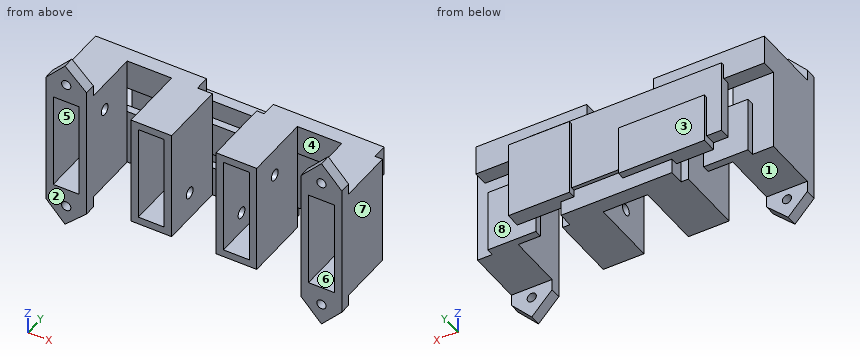
Autodesk Inventor part; units mm, degrees
ref_plane "Work Plane1" through (0, 18, 0) normal (0, 1, 0) x (-1, 0, 0)
ref_plane "YZ Plane" through (0, 0, 0) normal (1, 0, 0) x (0, 1, 0)
ref_plane "XY Plane" through (0, 0, 0) normal (0, 0, 1) x (1, 0, 0)
sketch "Sketch1" plane through (0, 0, 0) normal (0, 1, 0) x (-1, 0, 0)
  line L0 (0, 0) -> (80, 0) construction
  line L1 (80, 0) -> (80, 30) construction
  line L2 (80, 30) -> (0, 30) construction
  line L3 (0, 30) -> (0, 0) construction
  dimension "d0" = 80
  dimension "d1" = 30
sketch "Sketch2" plane through (0, 0, 0) normal (0, 1, 0) x (-1, 0, 0)
  line L0 (80, 0) -> (69, 0)
  line L1 (69, 0) -> (69, 30)
  line L2 (69, 30) -> (80, 30)
  line L3 (80, 30) -> (80, 0)
  line L4 (0, 0) -> (11, 0)
  line L5 (11, 0) -> (11, 30)
  line L6 (11, 30) -> (0, 30)
  line L7 (0, 30) -> (0, 0)
  line L8 (57, 0) -> (46, 0)
  line L9 (46, 0) -> (46, 30)
  line L10 (46, 30) -> (57, 30)
  line L11 (57, 30) -> (57, 0)
  line L12 (34, 0) -> (23, 0)
  line L13 (23, 0) -> (23, 30)
  line L14 (23, 30) -> (34, 30)
  line L15 (34, 30) -> (34, 0)
  line L16 (69, 15) -> (57, 15) construction
  line L17 (46, 15) -> (34, 15) construction
  line L18 (23, 15) -> (11, 15) construction
  line L19 (71, 2) -> (78, 2)
  line L20 (78, 2) -> (78, 28)
  line L21 (78, 28) -> (71, 28)
  line L22 (71, 28) -> (71, 2)
  line L23 (55, 2) -> (48, 2)
  line L24 (48, 2) -> (48, 28)
  line L25 (48, 28) -> (55, 28)
  line L26 (55, 28) -> (55, 2)
  line L27 (32, 2) -> (25, 2)
  line L28 (25, 2) -> (25, 28)
  line L29 (25, 28) -> (32, 28)
  line L30 (32, 28) -> (32, 2)
  line L31 (9, 28) -> (9, 2)
  line L32 (9, 2) -> (2, 2)
  line L33 (2, 2) -> (2, 28)
  line L34 (2, 28) -> (9, 28)
  dimension "d2" = 11
  dimension "d3" = 30
  dimension "d4" = 11
  dimension "d6" = 11
  dimension "d8" = 11
  dimension "d9" = 80
  dimension "d10" = 2
  dimension "d11" = 2
  dimension "d12" = 2
  dimension "d13" = 2
extrude "Extrusion1" add sketch "Sketch2" along normal blind 15
sketch "Sketch3" plane through (0, 15, 0) normal (0, 1, 0) x (1, 0, 0)
  line L0 (-69, 0) -> (-80, 0)
  line L1 (-80, 0) -> (-69, 0)
  line L2 (-69, 0) -> (-69, -30)
  line L3 (-69, -30) -> (-80, -30)
  line L4 (-80, -30) -> (-80, 0)
  line L5 (-57, 0) -> (-46, 0)
  line L6 (-46, 0) -> (-46, -30)
  line L7 (-46, -30) -> (-57, -30)
  line L8 (-57, -30) -> (-57, 0)
  line L9 (-34, 0) -> (-23, 0)
  line L10 (-23, 0) -> (-23, -30)
  line L11 (-23, -30) -> (-34, -30)
  line L12 (-34, -30) -> (-34, 0)
  line L13 (-11, 0) -> (0, 0)
  line L14 (0, 0) -> (0, -30)
  line L15 (0, -30) -> (-11, -30)
  line L16 (-11, -30) -> (-11, 0)
  dimension "d16" = 30
  dimension "d19" = 23
extrude "Extrusion2" add sketch "Sketch3" along normal blind 3
sketch "Sketch4" plane through (-69, 0, 30) normal (1, 0, 0) x (0, 0, -1)
  circle A0 centre (7.5, 8) radius 1.5
  line L0 (2, 0) -> (28, 0)
  line L1 (0, 0) -> (0, 18) construction
  dimension "d26" = 3
  dimension "d28" = 8
  dimension "d29" = 7.5
extrude "Extrusion3" cut sketch "Sketch4" against normal blind 3
sketch "Sketch5" plane through (-57, 0, 0) normal (-1, 0, 0) x (0, 0, 1)
  circle A0 centre (22.5, 8) radius 1.5
  line L0 (30, 0) -> (30, 18)
  line L1 (2, 0) -> (28, 0)
  point P0 (0, 0)
  dimension "d33" = 3
  dimension "d34" = 7.5
  dimension "d35" = 8
extrude "Extrusion4" cut sketch "Sketch5" against normal blind 3
sketch "Sketch6" plane through (-46, 0, 30) normal (1, 0, 0) x (0, 0, -1)
  circle A0 centre (22.5, 8) radius 1.5
  line L0 (30, 0) -> (30, 18)
  line L1 (2, 0) -> (28, 0)
  dimension "d38" = 3
  dimension "d39" = 7.5
  dimension "d40" = 8
sketch "Sketch7" plane through (-34, 0, 0) normal (-1, 0, 0) x (0, 0, 1)
  circle A0 centre (7.5, 8) radius 1.5
  line L0 (2, 0) -> (28, 0)
  line L1 (0, 0) -> (0, 18)
  dimension "d41" = 3
  dimension "d42" = 8
  dimension "d43" = 7.5
sketch "Sketch8" plane through (-23, 0, 30) normal (1, 0, 0) x (0, 0, -1)
  circle A0 centre (7.5, 8) radius 1.5
  line L0 (2, 0) -> (28, 0)
  line L1 (0, 0) -> (0, 18)
  point P0 (30, 0)
  dimension "d44" = 3
  dimension "d45" = 8
  dimension "d46" = 7.5
sketch "Sketch9" plane through (-11, 0, 0) normal (-1, 0, 0) x (0, 0, 1)
  point P0 (0, 0)
sketch "Sketch10" plane through (-11, 0, 0) normal (-1, 0, 0) x (0, 0, 1)
  circle A0 centre (22.5, 8) radius 1.5
  line L0 (30, 0) -> (30, 18)
  line L1 (2, 0) -> (28, 0)
  point P0 (0, 0)
  dimension "d47" = 3
  dimension "d48" = 7.5
  dimension "d49" = 8
extrude "Extrusion5" cut sketch "Sketch6" against normal blind 3
extrude "Extrusion6" cut sketch "Sketch7" against normal blind 3
extrude "Extrusion7" cut sketch "Sketch8" against normal blind 3
extrude "Extrusion8" cut sketch "Sketch10" against normal blind 3
ref_plane "Work Plane1" through (0, 18, 0) normal (0, 1, 0) x (-1, 0, 0)
sketch "Sketch12" plane through (0, 18, 0) normal (0, 1, 0) x (-1, 0, 0)
  line L0 (80, 30) -> (50, 30)
  line L1 (50, 30) -> (50, 22)
  line L2 (50, 22) -> (80, 22)
  line L3 (80, 22) -> (80, 30)
  line L4 (55, 0) -> (25, 0)
  line L5 (25, 0) -> (25, 8)
  line L6 (25, 8) -> (55, 8)
  line L7 (55, 8) -> (55, 0)
  line L8 (32, 2) -> (32, 28)
  line L9 (32, 22) -> (2, 22)
  line L10 (2, 22) -> (2, 30)
  line L11 (2, 30) -> (32, 30)
  line L12 (32, 30) -> (32, 22)
  point P0 (0, 0)
  dimension "d59" = 30
  dimension "d60" = 8
  dimension "d61" = 30
  dimension "d62" = 8
  dimension "d63" = 30
sketch "Sketch13" plane through (0, 18, 0) normal (0, 1, 0) x (-1, 0, 0)
  line L0 (74.3573, 0) -> (62.3573, 0)
  line L1 (62.3573, 0) -> (62.3573, 15)
  line L2 (62.3573, 15) -> (74.3573, 15)
  line L3 (74.3573, 15) -> (74.3573, 0)
  line L4 (48, 12) -> (36, 12)
  line L5 (36, 12) -> (36, 21)
  line L6 (36, 21) -> (48, 21)
  line L7 (48, 21) -> (48, 12)
  line L8 (0, 0) -> (11, 0)
  line L9 (4, 0) -> (17, 0)
  line L10 (17, 0) -> (17, 17)
  line L11 (17, 17) -> (4, 17)
  line L12 (4, 17) -> (4, 0)
  dimension "d64" = 12
  dimension "d65" = 15
  dimension "d66" = 12
  dimension "d67" = 13
  dimension "d68" = 17
extrude "Extrusion9" add sketch "Sketch13" along normal blind 2
extrude "Extrusion10" add sketch "Sketch12" along normal blind 4
sketch "Sketch14" plane through (0, 20, 0) normal (0, 1, 0) x (1, 0, 0)
  line L0 (-65, -4) -> (-41.7529, -4)
  line L1 (-41.7529, -4) -> (-41.7529, -17.4715)
  line L2 (-41.7529, -17.4715) -> (-65, -17.4715)
  line L3 (-65, -17.4715) -> (-65, -4)
  line L4 (-12, -25) -> (-28.5, -25)
  line L5 (-28.5, -25) -> (-28.5, -4)
  line L6 (-28.5, -4) -> (-12, -4)
  line L7 (-12, -4) -> (-12, -25)
  point P0 (0, 0)
  dimension "d73" = 16.5
extrude "Extrusion11" add sketch "Sketch14" along normal blind 4
sketch "Sketch15" plane through (0, 20, 0) normal (0, 1, 0) x (1, 0, 0)
  line L0 (-69, -30) -> (-69, -22)
  line L1 (-69, -26) -> (-17, -26)
  line L2 (-17, -26) -> (-17, -6)
  line L3 (-17, -6) -> (-69, -6)
  line L4 (-69, -6) -> (-69, -26)
  point P0 (0, 0)
  dimension "d76" = 52
  dimension "d77" = 20
extrude "Extrusion12" add sketch "Sketch15" along normal blind 3
sketch "Sketch16" plane through (0, 0, 0) normal (0, 1, 0) x (-1, 0, 0)
  line L0 (69, 30) -> (80, 30)
  line L1 (80, 30) -> (80, 33)
  line L2 (69, 30) -> (69, 33)
  line L3 (69, 33) -> (74.8182, 38.4908)
  line L4 (74.8182, 38.4908) -> (80, 33)
  circle A0 centre (74.5, 33) radius 1.25
  line L5 (74.5, 33) -> (80, 33) construction
  line L6 (74.5, 33) -> (69, 33) construction
  line L7 (11, 30) -> (11, 33)
  line L8 (0, 30) -> (0, 33)
  line L9 (11, 33) -> (5.5, 38.8095)
  line L10 (5.5, 38.8095) -> (0, 33)
  circle A1 centre (5.5, 33) radius 1.25
  line L11 (5.5, 33) -> (11, 33) construction
  line L12 (5.5, 33) -> (0, 33) construction
  line L13 (80, 15) -> (0, 15) construction
  line L14 (69, 0) -> (80, 0)
  line L15 (80, 0) -> (80, -3)
  line L16 (69, 0) -> (69, -3)
  line L17 (69, -3) -> (74.8182, -8.4908)
  line L18 (74.8182, -8.4908) -> (80, -3)
  circle A2 centre (74.5, -3) radius 1.25
  line L19 (74.5, -3) -> (80, -3) construction
  line L20 (74.5, -3) -> (69, -3) construction
  line L21 (11, 0) -> (11, -3)
  line L22 (0, 0) -> (0, -3)
  line L23 (11, -3) -> (5.5, -8.8095)
  line L24 (5.5, -8.8095) -> (0, -3)
  circle A3 centre (5.5, -3) radius 1.25
  line L25 (5.5, -3) -> (11, -3) construction
  line L26 (5.5, -3) -> (0, -3) construction
  line L27 (80, 0) -> (69, 0)
  line L28 (80, 0) -> (69, 0)
  line L29 (11, 0) -> (0, 0)
  line L30 (4, 0) -> (17, 0)
  line L31 (11, 30) -> (0, 30)
  dimension "d80" = 3
  dimension "d81" = 3
  dimension "d82" = 8
  dimension "d83" = 2.5
  dimension "d84" = 3
  dimension "d85" = 3
  dimension "d86" = 3
  dimension "d87" = 8
  dimension "d88" = 2.5
extrude "Extrusion14" add sketch "Sketch16" along normal blind 3
equation "\"d11\" = d10"
equation "\"d12\" = d10"
equation "\"d13\" = d10"
equation "\"d81\" = d80"
equation "\"d84\" = d81"
equation "\"d85\" = d86"
equation "\"d86\" = d84"
equation "\"d87\" = d82"
properties part number "ball-waterfall"
Part model, mm, in its own coordinate system. Face numbers are marked on the shaded views. A direction names the side the tool comes from. Round coordinates to 2 decimals unless told otherwise and drop trailing zeros. Order: outer loops, then holes, each group sorted by start corner. A loop starts at its lowest first (then second) coordinate and runs counter-clockwise, first axis right, second up. Notation, with made-up numbers: (-38.75, -39) -> (-25.75, -39) arc R30 cw to (-25.75, -3) -> close; hole circle Ø7 at (55, 84.25). An arc over 180 degrees is marked (long way). Put each result on its own line as item: value.
Q1. Band-saw the part on C-C (y = 8). State how many separate pieces and enclosed holes the cut face has, and give its area (3 significant figures).
From the geometry:
separate pieces: 6
enclosed holes: 0
area: 556 mm2
Q2. Band-saw the part on A-A (x = -37). Give the cut face in (y, z).
From the geometry:
outline: (18, 0) -> (22, 0) -> (22, 6) -> (23, 6) -> (23, 26) -> (20, 26) -> (20, 21) -> (18, 21) -> (18, 12) -> (20, 12) -> (20, 8) -> (18, 8) -> close
Q3. Pin check, flat tips, straight feed: pin 1 Ø10 at (x, y) = (-32.5, 9.5) entering from +Z; pin 2 Ø8.5 at (x, y) = (-10, 11.5) entering from -Z; pin 3 Ø8 at (x, z) = (-62, -1.5) entering from -Y. Stop position of each tip, or through.
From the geometry:
pin 1: stops at z = 30
pin 2: stops at z = 0
pin 3: stops at y = 18
Q4. Wall check: line 1 (Z direction, x = -5.5, y = 0.95); line 2 (Z direction, x = -31.5, y = 5.5); line 3 (Y direction, x = -23.7, z = 22.5). Give the ranges that are in metal, low to high. Write a range as [from, to].
From the geometry:
line 1: z = [-8.81, -4.25], [-1.75, 2], [28, 31.75], [34.25, 38.81]
line 2: z = [0, 2], [28, 30]
line 3: y = [0, 6.5], [9.5, 24]
Q5. Pull direction X, two halves, no side cores. Call the marked faces 6, 7 and 8: pulls with the +X half, pulls with the -X half, needs draft (parallel to the pull), parting line crosses it, or undercut.
From the geometry:
face 6: undercut
face 7: pulls with the +X half
face 8: needs draft
Q6. Band-saw the part on B-B (z = 35.5). Give the cut face in (x, y), and give its area (3 significant figures).
From the geometry:
outline: (-77.64, 0) -> (-71.65, 0) -> (-71.65, 3) -> (-77.64, 3) -> close; (-8.63, 0) -> (-2.37, 0) -> (-2.37, 3) -> (-8.63, 3) -> close
area: 36.8 mm2
Q7. Tool access for the marked faces 1, 2, 3, 4 and 5: list every direction of +Z, -Z, +X, -X, +Y, -Y with a clear straight run to the whole face (end or side of a thin tool).
From the geometry:
face 1: -Z, +X, -X, +Y
face 2: +Z, -Z, +X, -X, -Y
face 3: +Z, -Z, +X, -X, +Y
face 4: +Z, -Z, -Y
face 5: -Y
